Input: part model. Units: mm. Frame: model coordinates. A direction names the side the tool comes from. Give positions to 0.01 mm unless a question says otherwise; leave off trailing zeros. Write each loop counter-clockwise with the first axis right and the second up, starting at its lowest first coordinate (ties: lowest second). Pieces come first, ordered by that corner, then holes.
```python
from build123d import *

# Parameters (mm, degrees)
SKETCH_R          = 25.4
SKETCH_R_2        = 3.05
PAD_DEPTH         = 38.1
FILLET_R          = 0.5
SKETCH001_R       = 0.9
PAD001_DEPTH      = 19.05
PAD001_DEPTH_BACK = 3.5


with BuildPart() as fillet_body:
    # Sketch → Pad (new body)
    with BuildSketch(Plane.XY.offset(0.1)):
        with Locations((17.905, 0)):
            Circle(SKETCH_R)
        with Locations((17.905, 0)):
            Circle(SKETCH_R_2, mode=Mode.SUBTRACT)
    extrude(amount=PAD_DEPTH)

    # Fillet
    fillet_edges = [fillet_body.edges().sort_by_distance(p)[0] for p in [
        (14.855, 0, 38.2),
        (-7.495, 0, 38.2),
        (-7.495, 0, 0.1),
    ]]
    fillet(fillet_edges, radius=FILLET_R)


with BuildPart() as obj1:
    # Sketch001 → Pad001 (new body, two sides)
    with BuildSketch(Plane.XY.offset(0.5)) as pad001_sk:
        Circle(SKETCH001_R)
        with Locations((35.81, 0)):
            Circle(SKETCH001_R)
    extrude(amount=PAD001_DEPTH)
    extrude(pad001_sk.sketch, amount=-PAD001_DEPTH_BACK)

    # obj1: union Fillet body
    add(fillet_body.part)


solid = obj1.part
```
Item 1: Ray query, line 1 (Z direction, x = 37.5, y = 6); line 2 (Y direction, x = 19, z = 19.5); line 3 (Y direction, x = 8, z = 34.5). Return the intervals inside material, ascending.
Item 2: Mould query, pull axis X, two halves, no side actions, for faces 3 (the cylindrical face through (35.1, -0.55, -1.43)), 4 (the flat face through (23, 0, 38.2)), 5 (the cylindrical face through (42.13, 7.63, 18.89)). Classes: +X half, -X half, draft (parallel to the pull), parting line (faces both ways), or undercut.
Item 3: Section B-B (z = 3.5). Return loops of the section in (x, y) (3 decimals).
Item 4: Section A-A (y = 0). Return loops of the section in (x, z) (3 decimals).
Item 5: Set-up query: faces 1 (the flat face through (0, 0, -3)), 2 (the cylindrical face through (0.86, 0.27, -1.43)). Return all of +Z, -Z, +X, -X, +Y, -Y with unobstructed straight access to the full face (end or side cutting, diameter ignored); none if empty.
Item 6: Pin query (flat end, axial travel): pin 1 (2 mm diameter, centred on x = 20.5, z = 5, fed in from -Y); pin 2 (1 mm diameter, centred on x = 7.5, z = 5.5, fed in from +Y); pin 3 (1.5 mm diameter, centred on x = 22, z = 8.5, fed in from +Y). Return the tip coordinate at first contact, or that it passes through.
Solved:
1. line 1: z = 0.1 to 38.2
1. line 2: y = -25.38 to -2.85, 2.85 to 25.38
1. line 3: y = -23.39 to 23.39
2. face 3: undercut
2. face 4: draft
2. face 5: parting line
3. outline: circle Ø50.8 at (17.905, 0); hole circle Ø6.1 at (17.905, 0)
4. outline: (-7.495, 0.6) arc R0.5 ccw to (-6.995, 0.1) - (-0.9, 0.1) - (-0.9, -3) - (0.9, -3) - (0.9, 0.1) - (14.855, 0.1) - (14.855, 37.7) arc R0.5 ccw to (14.355, 38.2) - (-6.995, 38.2) arc R0.5 ccw to (-7.495, 37.7) - close; (20.955, 0.1) - (34.91, 0.1) - (34.91, -3) - (36.71, -3) - (36.71, 0.1) - (42.805, 0.1) arc R0.5 ccw to (43.305, 0.6) - (43.305, 37.7) arc R0.5 ccw to (42.805, 38.2) - (21.455, 38.2) arc R0.5 ccw to (20.955, 37.7) - close
5. face 1: -Z, +X, -X, +Y, -Y
5. face 2: -Z
6. pin 1: stops at y = -25.35
6. pin 2: stops at y = 23.39
6. pin 3: stops at y = 25.18
